Could you check a few things on this drawing? It's one solid part, dimensions in mm from its lowest x, y, z. Give positions to 0.01 mm unless a question says otherwise; leave off trailing zeros. Order: outer loops, then holes, each group sorted by start corner. A loop starts at its lowest first (then second) coordinate and runs counter-clockwise, first axis right, second up. Notation, with made-up numbers: (74.5, 79.5) - (126.5, 79.5) arc R22 ccw to (126.5, 101.5) - close; hole circle Ø8 at (62, -9.5). An arc over 180 degrees is marked (long way). Answer as CSV lines item,"result".
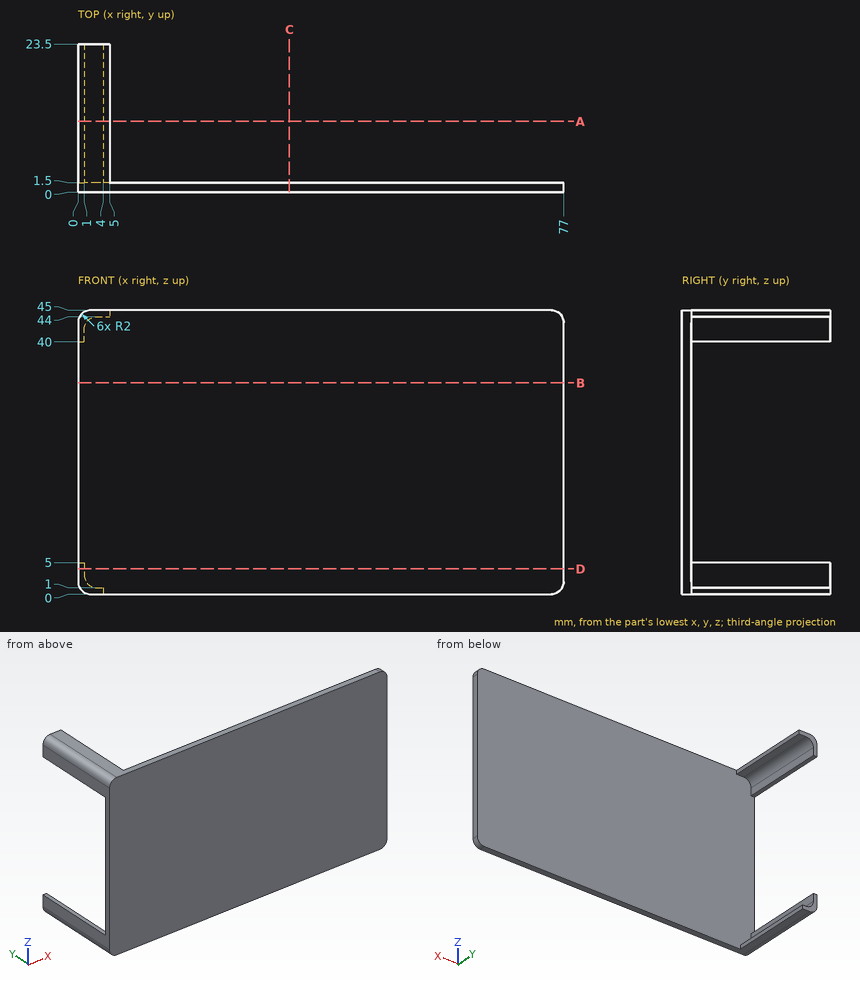
1) I want a section at C-C on x = 33.5. Write out the boundary of the cut face in (y, z), plus the area to 3 significant figures.
Answer block:
outline,"(0, 0) - (1.5, 0) - (1.5, 45) - (0, 45) - close"
area,"67.5 mm2"
2) I need wall thicknesses on line 1 along Y through (x, z) = (71, 32). Which ranges of the line are inside material? Lowest first, please. Write a range as [from, to].
Answer block:
line 1,"[0, 1.5]"
3) I want a section at D-D on z = 4. Write out the boundary of the cut face in (x, y), plus the area to 4 significant figures.
Answer block:
outline,"(0, 0) - (77, 0) - (77, 1.5) - (1, 1.5) - (1, 23.5) - (0, 23.5) - close"
area,"137.5 mm2"
4) I want a section at A-A on y = 11.25. Write out the boundary of the cut face in (x, z), plus the area to 3 significant figures.
Answer block:
outline,"(0, 2) arc R2 ccw to (2, 0) - (4, 0) - (4, 1) - (3, 1) arc R2 cw to (1, 3) - (1, 5) - (0, 5) - close; (0, 40) - (1, 40) - (1, 42) arc R2 cw to (3, 44) - (5, 44) - (5, 45) - (2, 45) arc R2 ccw to (0, 43) - close"
area,"17.0 mm2"
5) I'm going to push flat-ended pins straight in: P1, Ø10, axis at x = 49, z = 35, coming from the +Y side; P2, Ø1.1, axis at y = 11, z = 0.5, coming from the +X side; P3, Ø0.5, axis at x = 0.5, y = 9.5, coming from the +Z side; P4, Ø12, axis at y = 11, z = 27.5, coming from the +X side. Where does each tip first touch, or does it pass through?
Answer block:
P1,"y = 1.5"
P2,"x = 4"
P3,"z = 44.56"
P4,"through"
6) I want a section at B-B on z = 33.5. Write out the boundary of the cut face in (x, y).
Answer block:
outline,"(0, 0) - (77, 0) - (77, 1.5) - (0, 1.5) - close"
